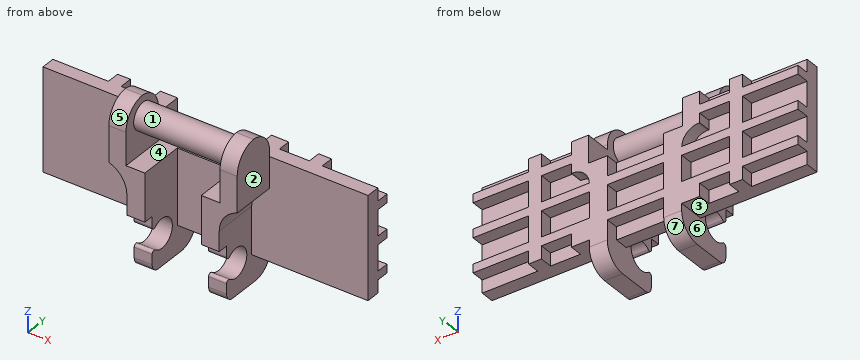
from build123d import *

# Parameters (mm, degrees)
SKETCH_1_W               = 38
SKETCH_1_H               = 12
EXTRUDE_1_DEPTH          = 1.6
EXTRUDE_START            = 1.6
SKETCH_1_3_W             = 38
SKETCH_1_3_H             = 1
SKETCH_1_3_W_2           = 1.5
SKETCH_1_3_H_2           = 12
EXTRUDE_2_DEPTH          = 1.5
EXTRUDE_START_2          = 3.1
EXTRUDE_3_DEPTH          = 8.4
SKETCH_2_4_W             = 2.1
SKETCH_2_4_H             = 1.5
EXTRUDE_5_DEPTH          = 3.1
CUT_EXTRUDE_1_DEPTH      = 22.850629282
FILLET_1_R               = 3
EXTRUDE_4_REACH          = 28.771
SKETCH_3_R               = 1.55
CUT_EXTRUDE_2_DEPTH      = 27.771253239
CUT_EXTRUDE_2_DEPTH_BACK = 27.771253239
SKETCH_3_3_R             = 1.7
SKETCH_3_3_W             = 6.5
SKETCH_3_3_H             = 1.2
SKETCH_3_3_W_2           = 3.4
SKETCH_3_3_H_2           = 3.1
FILLET_2_R               = 2.8
FILLET_3_R               = 2.5
FILLET_4_R               = 1
FILLET_5_R               = 0.3
FILLET_6_R               = 2


with BuildPart() as part:
    # 草图1 → 凸台-拉伸1 (new body)
    with BuildSketch(Plane(origin=(0, 0, 0), x_dir=(1, 0, 0), z_dir=(0, 1, 0))):
        Rectangle(SKETCH_1_W, SKETCH_1_H)
    extrude(amount=EXTRUDE_1_DEPTH)

    # 草图1<3> → 凸台-拉伸2 (add)
    with BuildSketch(Plane(origin=(0, 0, 0), x_dir=(1, 0, 0), z_dir=(0, 1, 0)).offset(EXTRUDE_START)):
        with Locations((0, 4)):
            Rectangle(SKETCH_1_3_W, SKETCH_1_3_H)
        Rectangle(SKETCH_1_3_W, SKETCH_1_3_H)
        with Locations((0, -4)):
            Rectangle(SKETCH_1_3_W, SKETCH_1_3_H)
        with Locations((-11.75, 0)):
            Rectangle(SKETCH_1_3_W_2, SKETCH_1_3_H_2)
        with Locations((11.75, 0)):
            Rectangle(SKETCH_1_3_W_2, SKETCH_1_3_H_2)
    extrude(amount=EXTRUDE_2_DEPTH)

    # 草图2 → 凸台-拉伸3 (add)
    with BuildSketch(Plane(origin=(0, 0, 0), x_dir=(1, 0, 0), z_dir=(0, 1, 0)).offset(EXTRUDE_START_2)):
        Polygon((-3.3, 9.3), (-5.4, 9.3), (-5.4, -2.4), (-7.5, -2.4), (-7.5, -9.4), (-5.5, -9.4), (-5.5, -2.8), (-3.3, -2.8), align=None)
        Polygon((5.4, 9.3), (3.3, 9.3), (3.3, -2.8), (5.5, -2.8), (5.5, -9.4), (7.5, -9.4), (7.5, -2.4), (5.4, -2.4), align=None)
    extrude(amount=-EXTRUDE_3_DEPTH)

    # 草图2<4> → 凸台-拉伸5 (add)
    with BuildSketch(Plane(origin=(0, 0, 0), x_dir=(1, 0, 0), z_dir=(0, 1, 0))):
        with Locations((-6.45, 5.25)):
            Rectangle(SKETCH_2_4_W, SKETCH_2_4_H)
        with Locations((6.45, 5.25)):
            Rectangle(SKETCH_2_4_W, SKETCH_2_4_H)
    extrude(amount=EXTRUDE_5_DEPTH)

    # 草图2<3> → 切除-拉伸1 (cut, through all)
    with BuildSketch(Plane(origin=(0, 0, 0), x_dir=(1, 0, 0), z_dir=(0, 1, 0))):
        Polygon((0, -9.4), (0, -2.8), (-3.3, -2.8), (-5.4, -2.8), (-5.5, -2.8), (-5.5, -9.4), align=None)
        Polygon((3.3, -2.8), (0, -2.8), (0, -9.4), (5.5, -9.4), (5.5, -2.8), (5.4, -2.8), align=None)
    extrude(amount=CUT_EXTRUDE_1_DEPTH, mode=Mode.SUBTRACT)

    # 圆角1
    # the kernel refuses this fillet: 3 mm, written as the material it adds along each edge
    with BuildSketch(Plane(origin=(5.4, 7.154544011, 2.4), x_dir=(1, 0, 0), z_dir=(0, -1, 0))) as fillet_1_piece_1_section:
        with BuildLine():
            CenterArc((3, -2.861817604), FILLET_1_R, 107.457603124, 72.542396876)
            Line((0, -2.861817604), (0, 0))
            Line((0, 0), (2.1, 0))
        make_face()
    fillet_1_piece_1 = extrude(amount=12.454544011, mode=Mode.PRIVATE)
    fillet_1_piece_1 = split(fillet_1_piece_1, bisect_by=Plane(origin=(6.297598678, 1.6, 1.686657362), z_dir=(0, -1, 0)), keep=Keep.TOP, mode=Mode.PRIVATE)
    add(fillet_1_piece_1)
    with BuildSketch(Plane(origin=(-5.4, 0, 2.4), x_dir=(0, 0, -1), z_dir=(0, -1, 0))) as fillet_1_piece_2:
        with BuildLine():
            CenterArc((2.861817604, -3), FILLET_1_R, 90, 72.542396876)
            Line((0, -2.1), (0, 0))
            Line((0, 0), (2.861817604, 0))
        make_face()
    extrude(amount=5.3)

    # 草图3 → 凸台-拉伸4 (add, up to next)
    with BuildSketch(Plane(origin=(-5.5, 0, 0), x_dir=(0, 0, -1), z_dir=(1, 0, 0)), mode=Mode.PRIVATE) as extrude_4_sk1:
        with Locations((-7, -2.5)):
            Circle(SKETCH_3_R)
    extrude_4_tool1 = extrude(extrude_4_sk1.sketch, amount=EXTRUDE_4_REACH, mode=Mode.PRIVATE) - part.part
    add(extrude_4_tool1.solids().sort_by_distance((-5.5, -2.5, 7))[0])

    # 草图3<3> → 切除-拉伸2 (cut, two sides: drawn at the far end of the back side and taken through both)
    with BuildSketch(Plane(origin=(-5.5, 0, 0), x_dir=(0, 0, -1), z_dir=(1, 0, 0)).offset(-CUT_EXTRUDE_2_DEPTH_BACK)):
        with Locations((5.58, -2.5)):
            Circle(SKETCH_3_3_R)
        with Locations((6.05, -4.7)):
            Rectangle(SKETCH_3_3_W, SKETCH_3_3_H)
        with Locations((-7.7, 1.55)):
            Rectangle(SKETCH_3_3_W_2, SKETCH_3_3_H_2)
    extrude(amount=CUT_EXTRUDE_2_DEPTH + CUT_EXTRUDE_2_DEPTH_BACK, mode=Mode.SUBTRACT)

    # 圆角2
    # the kernel refuses this fillet: 2.8 mm, written as the material it takes off along each edge
    with BuildSketch(Plane(origin=(-1.5, 0, 9.4), x_dir=(0, 0, -1), z_dir=(1, 0, 0)), Plane(origin=(-14.5, 0, 9.4), x_dir=(0, 0, -1), z_dir=(1, 0, 0))) as fillet_2_piece_1:
        with BuildLine():
            CenterArc((FILLET_2_R, -FILLET_2_R), FILLET_2_R, 90, 90)
            Line((0, -FILLET_2_R), (0, 0))
            Line((0, 0), (FILLET_2_R, 0))
        make_face()
    extrude(amount=16, mode=Mode.SUBTRACT)
    with BuildSketch(Plane(origin=(-1.5, -5.3, 9.4), x_dir=(0, 0, -1), z_dir=(1, 0, 0)), Plane(origin=(-14.5, -5.3, 9.4), x_dir=(0, 0, -1), z_dir=(1, 0, 0))) as fillet_2_piece_2:
        with BuildLine():
            CenterArc((FILLET_2_R, FILLET_2_R), FILLET_2_R, 180, 90)
            Line((0, FILLET_2_R), (0, 0))
            Line((0, 0), (FILLET_2_R, 0))
        make_face()
    extrude(amount=16, mode=Mode.SUBTRACT)

    # 圆角3
    fillet_3_edges = [part.edges().sort_by_distance(p)[0] for p in [
        (-4.35, 3.1, -9.3),
        (4.35, 3.1, -9.3),
    ]]
    fillet(fillet_3_edges, radius=FILLET_3_R)

    # 圆角4
    fillet_4_edges = [part.edges().sort_by_distance(p)[0] for p in [
        (-4.35, -4.1, -9.3),
        (4.35, -4.1, -9.3),
    ]]
    fillet(fillet_4_edges, radius=FILLET_4_R)

    # 圆角5
    fillet_5_edges = [part.edges().sort_by_distance(p)[0] for p in [
        (-4.35, -4.1, -5.005543735),
        (4.35, -4.1, -5.005543735),
        (-4.35, -4.1, -6.154456265),
        (4.35, -4.1, -6.154456265),
    ]]
    fillet(fillet_5_edges, radius=FILLET_5_R)

    # 圆角6
    # the kernel refuses this fillet: 2 mm, written as the material it adds along each edge
    with BuildSketch(Plane(origin=(5.4, 3.1, 2.4), x_dir=(0, 0, -1), z_dir=(0, -1, 0))) as fillet_6_piece_1:
        with BuildLine():
            CenterArc((2, 1.997498436), FILLET_6_R, 180, 87.134016017)
            Line((0, 1.997498436), (-0.04, 1.997498436))
            Line((-0.04, 1.997498436), (-0.04, 0))
            Line((-0.04, 0), (0, -0.04))
            ThreePointArc((0, -0.04), (0.95, -0.04), (1.898, -0.039949969))
            Line((1.898, -0.039949969), (1.9, 0))
        make_face()
    extrude(amount=6.493746089)
    with BuildSketch(Plane(origin=(-5.4, 3.1, 2.4), x_dir=(-1, 0, 0), z_dir=(0, -1, 0))) as fillet_6_piece_2:
        with BuildLine():
            CenterArc((1.997498436, 2), FILLET_6_R, 182.865983983, 87.134016017)
            Line((0, 1.9), (-0.039949969, 1.898))
            ThreePointArc((-0.039949969, 1.898), (-0.04, 0.95), (-0.04, 0))
            Line((-0.04, 0), (0, -0.04))
            Line((0, -0.04), (1.997498436, -0.04))
            Line((1.997498436, -0.04), (1.997498436, 0))
        make_face()
    extrude(amount=6.493746089)


solid = part.part
Could you check a few things on this model? Use its own coordinates, in mm. Face numbers are marked on the shaded views. A direction names the side the tool comes from. Round coordinates to 2 decimals unless told otherwise and drop trailing zeros. Write each loop counter-clockwise with the first axis right and the second up, starting at its lowest first coordinate (ties: lowest second). Pieces come first, ordered by that corner, then holes. Notation, with made-up numbers: (-8.75, -29) -> (44.25, -29) arc R26 cw to (44.25, -7) -> close; hole circle Ø6 at (-28.75, 38.25). An arc over 180 degrees is marked (long way). Use a Markdown table: item, result.
1. Please list where these lines run through material, in increasing order: probe 1 along X at (y, z) = (2.5, -1); probe 2 along Z at (x, y) = (4.5, -2.5); probe 3 along Z at (x, y) = (15.5, 2.25).
Answer key:
| item | result |
|---|---|
| probe 1 | x = -12.5 to -11, -5.4 to -3.3, 3.3 to 5.4, 11 to 12.5 |
| probe 2 | z = -9.3 to -7.28, -3.88 to 2.8, 5.45 to 8.55 |
| probe 3 | z = -4.5 to -3.5, -0.5 to 0.5, 3.5 to 4.5 |
2. If we section it at B-B (z = -5.58): List the corners of the cut face in (x, y) for me.
Answer key:
| item | result |
|---|---|
| outline | (-19, 0) -> (-5.4, 0) -> (-5.4, -0.8) -> (-3.3, -0.8) -> (-3.3, 0) -> (3.3, 0) -> (3.3, -0.8) -> (5.4, -0.8) -> (5.4, 0) -> (19, 0) -> (19, 1.6) -> (12.5, 1.6) -> (12.5, 3.1) -> (11, 3.1) -> (11, 1.6) -> (7.5, 1.6) -> (7.5, 3.1) -> (3.3, 3.1) -> (3.3, 1.6) -> (-3.3, 1.6) -> (-3.3, 3.1) -> (-7.5, 3.1) -> (-7.5, 1.6) -> (-11, 1.6) -> (-11, 3.1) -> (-12.5, 3.1) -> (-12.5, 1.6) -> (-19, 1.6) -> close |
3. If we section it at C-C (x = -15.5): List the corners of the cut face in (y, z) for me, then the cut area to 3 significant figures.
Answer key:
| item | result |
|---|---|
| outline | (0, -6) -> (1.6, -6) -> (1.6, -4.5) -> (3.1, -4.5) -> (3.1, -3.5) -> (1.6, -3.5) -> (1.6, -0.5) -> (3.1, -0.5) -> (3.1, 0.5) -> (1.6, 0.5) -> (1.6, 3.5) -> (3.1, 3.5) -> (3.1, 4.5) -> (1.6, 4.5) -> (1.6, 6) -> (0, 6) -> close |
| area | 23.7 mm^2 |
4. Which directions (+Z, -Z, +X, -X, +Y, -Y) give clear straight access to the entire face, cutting with the end or side of a thin tool? Please do the marked faces 1, 2 and 3.
Answer key:
| item | result |
|---|---|
| face 1 | none |
| face 2 | +Z, -Z, +X, -Y |
| face 3 | -Z, -X, +Y, -Y |
5. We'd pull the mould along Z, two halves only. Please class the marked faces 4, 5, 6 and 7: +Z half, -Z half, draft (parallel to the pull), parting line (faces both ways), or undercut.
Answer key:
| item | result |
|---|---|
| face 4 | undercut |
| face 5 | +Z half |
| face 6 | draft |
| face 7 | -Z half |
6. For pin 1 Ø2 at (y, z) = (-1.5, 7.5) entering from -X; pin 2 Ø1.6 at (x, y) = (16, 2) entering from +Z; pin 3 Ø9.5 at (x, z) = (-11.5, -2.5) entering from -Y, each with a flat end and sliding along its axis, tell me the tip position at first contact or that it passes through.
Answer key:
| item | result |
|---|---|
| pin 1 | stops at x = -7.5 |
| pin 2 | stops at z = 6 |
| pin 3 | stops at y = 0 |
7. If we section it at A-A (x = 0): List the corners of the cut face in (y, z) for me.
Answer key:
| item | result |
|---|---|
| outline | circle Ø3.1 at (-2.5, 7); (0, -6) -> (1.6, -6) -> (1.6, -4.5) -> (3.1, -4.5) -> (3.1, -3.5) -> (1.6, -3.5) -> (1.6, -0.5) -> (3.1, -0.5) -> (3.1, 0.5) -> (1.6, 0.5) -> (1.6, 2.8) -> (0, 2.8) -> close |
8. If we section it at D-D (y = -1.75): List the corners of the cut face in (x, z) for me, then the cut area to 3 significant figures.
Answer key:
| item | result |
|---|---|
| outline | (-7.5, 2.4) arc R3 cw to (-5.4, -0.46) -> (-5.4, -4.05) -> (-3.3, -4.05) -> (-3.3, 2.8) -> (-5.5, 2.8) -> (-5.5, 5.64) -> (5.5, 5.64) -> (5.5, 2.8) -> (3.3, 2.8) -> (3.3, -4.05) -> (5.4, -4.05) -> (5.4, -0.46) arc R3 cw to (7.5, 2.4) -> (7.5, 9.2) -> (5.5, 9.2) -> (5.5, 8.36) -> (-5.5, 8.36) -> (-5.5, 9.2) -> (-7.5, 9.2) -> close; (-5.4, -9.3) -> (-3.3, -9.3) -> (-3.3, -7.11) -> (-5.4, -7.11) -> close; (3.3, -9.3) -> (5.4, -9.3) -> (5.4, -7.11) -> (3.3, -7.11) -> close |
| area | 98.3 mm^2 |
